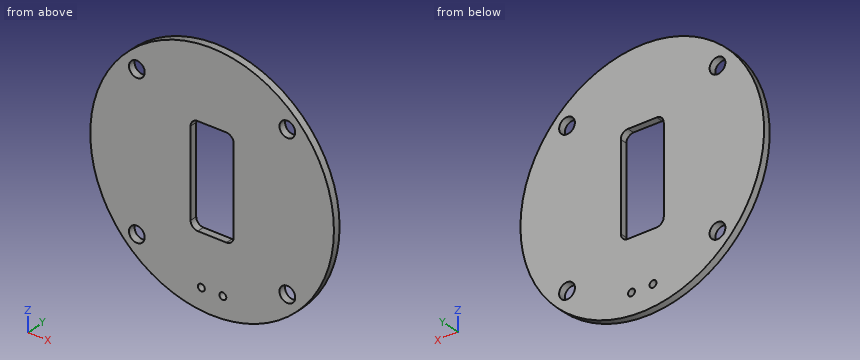
```python
from build123d import *

# Parameters (mm, degrees)
SKETCH1_R          = 85
BASE_DEPTH         = 5
BOLT_HOLES_REACH   = 7
SKETCH2_R          = 5.5
SLOT_REACH         = 7
SKETCH5_R          = 2.4
SWITCH_HOLES_DEPTH = 5


with BuildPart() as part:
    # Sketch1 → Base (new body)
    with BuildSketch(Plane(origin=(0, 0, 0), x_dir=(1, 0, 0), z_dir=(0, 1, 0))):
        Circle(SKETCH1_R)
    extrude(amount=BASE_DEPTH)

    # Sketch2 → Bolt Holes (cut, up to next)
    with BuildSketch(Plane(origin=(0, 5, 0), x_dir=(1, 0, 0), z_dir=(0, 1, 0)), mode=Mode.PRIVATE) as bolt_holes_sk1:
        with Locations((52.5, 52.5)):
            Circle(SKETCH2_R)
    bolt_holes_tool1 = extrude(bolt_holes_sk1.sketch, amount=-BOLT_HOLES_REACH, mode=Mode.PRIVATE) & part.part
    add(bolt_holes_tool1.solids().sort_by_distance((52.5, 5, -52.5))[0], mode=Mode.SUBTRACT)
    # Sketch2 → Bolt Holes (cut, up to next)
    with BuildSketch(Plane(origin=(0, 5, 0), x_dir=(1, 0, 0), z_dir=(0, 1, 0)), mode=Mode.PRIVATE) as bolt_holes_sk2:
        with Locations((-52.5, 52.5)):
            Circle(SKETCH2_R)
    bolt_holes_tool2 = extrude(bolt_holes_sk2.sketch, amount=-BOLT_HOLES_REACH, mode=Mode.PRIVATE) & part.part
    add(bolt_holes_tool2.solids().sort_by_distance((-52.5, 5, -52.5))[0], mode=Mode.SUBTRACT)
    # Sketch2 → Bolt Holes (cut, up to next)
    with BuildSketch(Plane(origin=(0, 5, 0), x_dir=(1, 0, 0), z_dir=(0, 1, 0)), mode=Mode.PRIVATE) as bolt_holes_sk3:
        with Locations((52.5, -52.5)):
            Circle(SKETCH2_R)
    bolt_holes_tool3 = extrude(bolt_holes_sk3.sketch, amount=-BOLT_HOLES_REACH, mode=Mode.PRIVATE) & part.part
    add(bolt_holes_tool3.solids().sort_by_distance((52.5, 5, 52.5))[0], mode=Mode.SUBTRACT)
    # Sketch2 → Bolt Holes (cut, up to next)
    with BuildSketch(Plane(origin=(0, 5, 0), x_dir=(1, 0, 0), z_dir=(0, 1, 0)), mode=Mode.PRIVATE) as bolt_holes_sk4:
        with Locations((-52.5, -52.5)):
            Circle(SKETCH2_R)
    bolt_holes_tool4 = extrude(bolt_holes_sk4.sketch, amount=-BOLT_HOLES_REACH, mode=Mode.PRIVATE) & part.part
    add(bolt_holes_tool4.solids().sort_by_distance((-52.5, 5, 52.5))[0], mode=Mode.SUBTRACT)

    # Sketch4 → Slot (cut, up to next)
    with BuildSketch(Plane(origin=(0, 5, 0), x_dir=(1, 0, 0), z_dir=(0, 1, 0)), mode=Mode.PRIVATE) as slot_sk1:
        with BuildLine():
            Line((10, -35), (-10, -35))
            ThreePointArc((-10, -35), (-13.535533906, -33.535533906), (-15, -30))
            Line((-15, -30), (-15, 30))
            ThreePointArc((-15, 30), (-13.535533906, 33.535533906), (-10, 35))
            Line((-10, 35), (10, 35))
            ThreePointArc((10, 35), (13.535533906, 33.535533906), (15, 30))
            Line((15, 30), (15, -30))
            ThreePointArc((15, -30), (13.535533906, -33.535533906), (10, -35))
        make_face()
    slot_tool1 = extrude(slot_sk1.sketch, amount=-SLOT_REACH, mode=Mode.PRIVATE) & part.part
    add(slot_tool1.solids().sort_by_distance((0, 5, 0))[0], mode=Mode.SUBTRACT)

    # Sketch5 → Switch Holes (cut)
    with BuildSketch(Plane(origin=(0, 5, 0), x_dir=(1, 0, 0), z_dir=(0, 1, 0))):
        with Locations((7.5, 70)):
            Circle(SKETCH5_R)
        with Locations((-7.5, 70)):
            Circle(SKETCH5_R)
    extrude(amount=-SWITCH_HOLES_DEPTH, mode=Mode.SUBTRACT)


solid = part.part
```
Can you work these out from the model? Positions are in its coordinate system, mm. Give positions to 0.01 mm unless a question says otherwise; leave off trailing zeros. Write each loop counter-clockwise with the first axis right and the second up, starting at its lowest first coordinate (ties: lowest second). Pieces come first, ordered by that corner, then holes. Notation, with made-up numbers: (-20.5, 83.5) - (8.5, 83.5) arc R19 cw to (8.5, 95.5) - close; hole circle Ø6 at (39.5, 80.5). An arc over 180 degrees is marked (long way). Write item = value, one per line. Start each with the question number.
1. For pin 1 (2 mm diameter, centred on y = 3.5, z = 29, fed in from +X); pin 2 (3 mm diameter, centred on x = 65, z = 12.5, fed in from -Y); pin 3 (9 mm diameter, centred on x = 52.5, z = -52.5, fed in from +Y); pin 4 (3 mm diameter, centred on y = 0.5, z = -63, fed in from -X), each with a flat end and sliding along its axis, tell me the tip position at first contact or that it passes through.
2. Please list where these lines run through material, in increasing order: line 1 (Z direction, x = -52.5, y = 3.3); line 2 (X direction, y = 3.9, z = -50).
3. Imagine slicing it at C-C (y = 1.25). Please give me the cut outline in (x, z), and give its area (3 significant figures).
4. Imagine slicing it at B-B (z = 0). Please give me the cut outline in (x, y).
5. Imagine slicing it at A-A (x = 0). Please give me the cut outline in (y, z), and give its area (3 significant figures).
6. Imagine slicing it at D-D (z = 52.5). Please give me the cut outline in (x, y).
Worked answers:
q1.pin_1 = 80.26
q1.pin_2 = 0
q1.pin_3 = through
q1.pin_4 = -58.67
q2.line_1 = -66.85 to -58, -47 to 47, 58 to 66.85
q2.line_2 = -68.74 to -57.4, -47.6 to 47.6, 57.4 to 68.74
q3.outline = circle Ø170 at (0, 0); hole circle Ø11 at (-52.5, -52.5); hole circle Ø11 at (-52.5, 52.5); hole (-15, -30) arc R5 ccw to (-10, -35) - (10, -35) arc R5 ccw to (15, -30) - (15, 30) arc R5 ccw to (10, 35) - (-10, 35) arc R5 ccw to (-15, 30) - close; hole circle Ø4.8 at (-7.5, -70); hole circle Ø4.8 at (7.5, -70); hole circle Ø11 at (52.5, -52.5); hole circle Ø11 at (52.5, 52.5)
q3.area = 20,200 mm2
q4.outline = (-85, 0) - (-15, 0) - (-15, 5) - (-85, 5) - close; (15, 0) - (85, 0) - (85, 5) - (15, 5) - close
q5.outline = (0, -85) - (5, -85) - (5, -35) - (0, -35) - close; (0, 35) - (5, 35) - (5, 85) - (0, 85) - close
q5.area = 500 mm2
q6.outline = (-66.85, 0) - (-58, 0) - (-58, 5) - (-66.85, 5) - close; (-47, 0) - (47, 0) - (47, 5) - (-47, 5) - close; (58, 0) - (66.85, 0) - (66.85, 5) - (58, 5) - close
